The model under review builds one solid part; all positions refer to its coordinate system, in mm. A direction names the side the tool comes from. Coordinates: 2 decimals unless noted, no trailing zeros. Write each loop counter-clockwise with the first axis right and the second up, starting at its lowest first coordinate (ties: lowest second). Pieces come first, ordered by that corner, then holes. Notation, with made-up numbers: M -35.5,62 L -8.5,62 A21 ccw -8.5,93 Z; hole C -7,6.25 d8. An arc over 180 degrees is marked long. Answer as CSV lines item,"result". Start each with the question number.
Autodesk Inventor part; units mm, degrees
ref_plane "YZ Plane" through (0, 0, 0) normal (1, 0, 0) x (0, 1, 0)
ref_plane "XZ Plane" through (0, 0, 0) normal (0, 1, 0) x (-1, 0, 0)
ref_plane "XY Plane" through (0, 0, 0) normal (0, 0, 1) x (1, 0, 0)
sketch "Skizze1" plane through (0, 0, 0) normal (0, 1, 0) x (-1, 0, 0)
  line L0 (0, 0) -> (140, 0)
  line L1 (140, 0) -> (140, -45)
  line L2 (140, -45) -> (0, -45)
  line L3 (0, -45) -> (0, 0)
  dimension "d0" = 140
  dimension "d1" = 45
extrude "Extrusion1" add sketch "Skizze1" along normal blind 18
sketch "Skizze2" plane through (0, 18, 0) normal (0, 1, 0) x (1, 0, 0)
  line L0 (0, 0) -> (0, 45)
  line L1 (0, 45) -> (-140, 45)
  line L2 (-140, 45) -> (-140, 0)
  point P0 (-131, 35)
  point P1 (-131, 10)
  point P2 (-9, 35)
  point P3 (-9, 10)
  dimension "d14" = 10
  dimension "d15" = 25
  dimension "d16" = 10
  dimension "d17" = 25
  dimension "d18" = 9
  dimension "d19" = 9
hole "Bohrung1" at (-131, 18, -35) at (-131, 18, -10) at (-9, 18, -35) at (-9, 18, -10) direction (0, -1, 0) diameter 2 end through all countersink diameter 5 countersink angle 90
fillet "Rundung3" radius 5 2 edges at (0, 18, -22.5) (-140, 18, -22.5)
sketch "Skizze3" plane through (0, 18, 0) normal (0, 1, 0) x (1, 0, 0)
  line L0 (-135, 0) -> (-5, 0)
  line L1 (-35, 15) -> (-52, 15)
  line L2 (-52, 15) -> (-52, 30)
  line L3 (-52, 30) -> (-35, 30)
  line L4 (-35, 30) -> (-35, 15)
  line L5 (0, 0) -> (0, 45)
  line L6 (-140, 45) -> (-140, 0)
  circle A0 centre (-100, 22.5) radius 2.5
  dimension "d32" = 17
  dimension "d33" = 15
  dimension "d34" = 15
  dimension "d39" = 35
  dimension "d40" = 5
  dimension "d41" = 22.5
  dimension "d42" = 40
extrude "Extrusion3" cut sketch "Skizze3" against normal blind 18
properties part number "Seitenteil_mit_Sensoren" material "Eiche, weiß"
1) Mouldability with a two-part tool opening along X and no side actions: class faces 3 (the cylindrical face through (-139, 16, -23)), 4 (the flat face through (-69, 0, -22)), 5 (the flat face through (-43, 9, -15)) as +X half, -X half, draft (parallel to the pull), parting line (faces both ways), or undercut.
2) Clearance check with flat-ended pins moving along their axes: pin 1 Ø1.8 at (x, z) = (-131, -10) entering from -Y; pin 2 Ø5 at (x, y) = (-45, 4.5) entering from +Z; pin 3 Ø2.5 at (x, z) = (-131, -35) entering from +Y. State where each tip first meets the part, or that it passes through.
3) To check wall thickness, follow line 1 (X direction, y = 7, z = -10); line 2 (X direction, y = 10.25, z = -22.5); line 3 (Z direction, x = -131, y = 6.75). State the ranges of each line that lie inside material, in increasing order. Write a range as [from, to].
4) Tool access review of faces 1 (the cylindrical face through (-1, 16, -22)), 2 (the flat face through (-52, 9, -22)): name each direction out of +Z, -Z, +X, -X, +Y, -Y from which nothing blocks a thin tool from reaching the whole face with its end or side.
5) Take a section at D-D on x = -100. Give the boundary of the cut face in (y, z).
6) Take a section at C-C on y = 4.25. Give the boundary of the cut face in (x, z).
7) Take a section at A-A on x = -37. Give the boundary of the cut face in (y, z).
8) Take a section at B-B on z = -22.5. Give the boundary of the cut face in (x, y).
Results:
1,face 3,"-X half"
1,face 4,"draft"
1,face 5,"undercut"
2,pin 1,"passes through"
2,pin 2,"stops at z = 0"
2,pin 3,"stops at y = 16.75"
3,line 1,"x = [-140, -132], [-130, -10], [-8, 0]"
3,line 2,"x = [-140, -102.5], [-97.5, -52], [-35, 0]"
3,line 3,"z = [-45, -36], [-34, -11], [-9, 0]"
4,face 1,"+Z, -Z, +X, +Y"
4,face 2,"+Y, -Y"
5,outline,"M 0,-45 L 18,-45 L 18,-25 L 0,-25 Z; M 0,-20 L 18,-20 L 18,0 L 0,0 Z"
6,outline,"M -140,-45 L 0,-45 L 0,0 L -140,0 Z; hole C -131,-35 d2; hole C -131,-10 d2; hole C -100,-22.5 d5; hole M -52,-30 L -35,-30 L -35,-15 L -52,-15 Z; hole C -9,-35 d2; hole C -9,-10 d2"
7,outline,"M 0,-45 L 18,-45 L 18,-30 L 0,-30 Z; M 0,-15 L 18,-15 L 18,0 L 0,0 Z"
8,outline,"M -140,0 L -102.5,0 L -102.5,18 L -135,18 A5 ccw -140,13 Z; M -97.5,0 L -52,0 L -52,18 L -97.5,18 Z; M -35,0 L 0,0 L 0,13 A5 ccw -5,18 L -35,18 Z"
